The listing builds one solid part. Answer for the finished solid, in the listing's coordinates (mm). A direction names the side the tool comes from. Coordinates: 2 decimals unless noted, no trailing zeros. Write each loop counter-clockwise with the first axis right and the second up, starting at its lowest first coordinate (ties: lowest second). Pieces come first, ordered by that corner, then holes.
(1) Given P1, Ø1.5, axis at y = 30, z = 1, coming from the +X side, flat-ended and moving along its own axis, determine where the tip first touches the part or whether it passes through.
(2) Which of the six approach directions +Z, -Z, +X, -X, +Y, -Y give full straight-line access (tool end or side, diameter ignored) to faces 1 (the flat face through (3, 0, 1)), 2 (the flat face through (5, 24, 1)), 3 (the flat face through (11.471, 52.455, 1.479)), 4 (the flat face through (5, 55, 1))?
(3) The part is cut by section C-C on y = 39. Determine the outline of the cut face in (x, z), plus the area to 3 significant figures.
(4) The part is cut by section A-A on y = 86.5. Determine the outline of the cut face in (x, z).
(5) The part is cut by section B-B on z = 0.95. Determine the outline of the cut face in (x, y) (1 decimal).
(6) Straight lines are drawn through the part: line 1 (X direction, y = 6.5, z = 1.8); line 2 (Y direction, x = 8, z = 2.4); line 3 (X direction, y = 63, z = 1.4). For each, find the intervals that lie inside material, in ascending order.
(7) For a pull along X with two mould halves and no side action, classify faces 5 (the flat face through (15.447, 79.636, 1.479)), 6 (the cylindrical face through (7.388, 95.977, 1.479)), 7 (the cylindrical face through (18.514, 60.989, 1.479)) as +X half, -X half, draft (parallel to the pull), parting line (faces both ways), or undercut.
(8) The part is cut by section D-D on y = 74. Determine the outline of the cut face in (x, z).
from build123d import *

# Parameters (mm, degrees)
PAD_DEPTH    = 3
POCKET_DEPTH = 3.001


with BuildPart() as part:
    # Sketch → Pad (new body)
    with BuildSketch(Plane.XY):
        with BuildLine():
            Line((0, 0), (0, 88))
            ThreePointArc((15.849182, 89.546106), (7.223278, 95.962235), (0, 88))
            Line((15.849182, 89.546106), (19, 70))
            ThreePointArc((14.497745, 53.183248), (18.54727, 61.110149), (19, 70))
            Line((14.497745, 53.183248), (10.641979, 50))
            Line((10.641979, 50), (10, 50.47735))
            Line((10, 50.47735), (12.983436, 54.48972))
            ThreePointArc((12.983436, 54.48972), (16.50721, 61.852406), (17, 70))
            Line((17, 70), (13.849182, 89.546106))
            ThreePointArc((13.849182, 89.546106), (7.174445, 94.522086), (2, 88))
            Line((2, 88), (5, 58))
            Line((5, 58), (5, 0))
            Line((5, 0), (0, 0))
        make_face()
    extrude(amount=PAD_DEPTH)

    # Sketch001 → Pocket (cut, through all)
    with BuildSketch(Plane.XY.offset(3)):
        with BuildLine():
            ThreePointArc((5, 52), (3, 49.5), (5, 47))
            Line((5, 52), (5, 47))
        make_face()
    extrude(amount=-POCKET_DEPTH, mode=Mode.SUBTRACT)


solid = part.part
Model answer:
1. P1: stops at x = 5
2. face 1: +Z, -Z, +X, -X, -Y
2. face 2: +Z, -Z, +X, -Y
2. face 3: +Z, -Z
2. face 4: +Z, -Z, -Y
3. outline: (0, 0) - (5, 0) - (5, 3) - (0, 3) - close
3. area: 15.0 mm2
4. outline: (0, 0) - (2.15, 0) - (2.15, 3) - (0, 3) - close; (14.34, 0) - (16.34, 0) - (16.34, 3) - (14.34, 3) - close
5. outline: (0, 0) - (5, 0) - (5, 47) arc R2.6 cw to (5, 52) - (5, 58) - (2, 88) arc R6 cw to (13.8, 89.5) - (17, 70) arc R21.3 cw to (13, 54.5) - (10, 50.5) - (10.6, 50) - (14.5, 53.2) arc R21.3 ccw to (19, 70) - (15.8, 89.5) arc R8 ccw to (0, 88) - close
6. line 1: x = 0 to 5
6. line 2: y = 94.57 to 96
6. line 3: x = 0 to 4.5, 16.77 to 18.96
7. face 5: undercut
7. face 6: parting line
7. face 7: +X half
8. outline: (0, 0) - (3.4, 0) - (3.4, 3) - (0, 3) - close; (16.36, 0) - (18.36, 0) - (18.36, 3) - (16.36, 3) - close
